```python
from build123d import *

# Parameters (mm, degrees)
SKETCH1_W           = 220
SKETCH1_H           = 30
BOSS_EXTRUDE1_DEPTH = 5
SKETCH2_W           = 30
SKETCH2_H           = 70
BOSS_EXTRUDE2_DEPTH = 5
CUT_EXTRUDE1_DEPTH  = 10
BOSS_EXTRUDE3_DEPTH = 5
BOSS_EXTRUDE4_DEPTH = 30
FILLET1_R           = 5
SKETCH7_R           = 7.5
CUT_EXTRUDE2_DEPTH  = 253
SKETCH8_W           = 15
SKETCH8_H           = 14.618243145
BOSS_EXTRUDE5_DEPTH = 5
FILLET2_R           = 5
CUT_EXTRUDE3_DEPTH  = 5
SKETCH10_W          = 5.944140112
SKETCH10_H          = 11.167837108
SKETCH10_W_2        = 5.92832961
SKETCH10_H_2        = 9.506983552
CUT_EXTRUDE4_DEPTH  = 5
SKETCH11_W          = 5.623434756
SKETCH11_H          = 8.337110403
SKETCH11_W_2        = 5.64698147
SKETCH11_H_2        = 9.10404701
CUT_EXTRUDE5_DEPTH  = 5
FILLET3_R           = 1
CUT_EXTRUDE6_DEPTH  = 5
SKETCH13_W          = 6.176524638
SKETCH13_H          = 11.481735796
SKETCH13_W_2        = 6.413794009
SKETCH13_H_2        = 10.832022022
CUT_EXTRUDE7_DEPTH  = 5


with BuildPart() as part:
    # Sketch1 → Boss-Extrude1 (new body)
    with BuildSketch(Plane(origin=(0, 0, 0), x_dir=(1, 0, 0), z_dir=(0, 1, 0))):
        Rectangle(SKETCH1_W, SKETCH1_H)
    extrude(amount=BOSS_EXTRUDE1_DEPTH)

    # Sketch2 → Boss-Extrude2 (add)
    with BuildSketch(Plane.ZY.offset(110)):
        with Locations((0, -30)):
            Rectangle(SKETCH2_W, SKETCH2_H)
    boss_extrude2 = extrude(amount=BOSS_EXTRUDE2_DEPTH)

    # Mirror1: Boss-Extrude2 across plane
    add(boss_extrude2.mirror(Plane(origin=(0, 0, 0), x_dir=(0, 0, 1), z_dir=(1, 0, 0))))

    # Sketch4 → Cut-Extrude1 (cut)
    with BuildSketch(Plane.ZY.offset(115)):
        with BuildLine():
            Line((-15, -47.167473829), (-15, -65))
            Line((-15, -65), (15, -65))
            Line((15, -65), (15, -47.167473829))
            ThreePointArc((15, -47.167473829), (0, -62.167473829), (-15, -47.167473829))
        make_face()
    cut_extrude1 = extrude(amount=-CUT_EXTRUDE1_DEPTH, mode=Mode.SUBTRACT)

    # Mirror2: Cut-Extrude1 across plane
    add(cut_extrude1.mirror(Plane(origin=(0, 0, 0), x_dir=(0, 0, 1), z_dir=(1, 0, 0))), mode=Mode.SUBTRACT)

    # Sketch5 → Boss-Extrude3 (add)
    with BuildSketch(Plane(origin=(115, 0, 0), x_dir=(0, 0, -1), z_dir=(1, 0, 0))):
        with BuildLine():
            Line((28.523256762, -29.22115135), (15, -31.288780588))
            Line((15, -31.288780588), (-5.201478884, -40.890888071))
            Line((-5.201478884, -40.890888071), (-4.123987776, -59.07486744))
            Line((-4.123987776, -59.07486744), (0, -62.167473829))
            ThreePointArc((0, -62.167473829), (7.341637998, -60.248007132), (12.804338712, -54.98085403))
            Line((12.804338712, -54.98085403), (28.523256762, -29.22115135))
        make_face()
    boss_extrude3 = extrude(amount=-BOSS_EXTRUDE3_DEPTH)

    # Mirror3: Boss-Extrude3 across plane
    add(boss_extrude3.mirror(Plane(origin=(0, 0, 0), x_dir=(0, 0, 1), z_dir=(1, 0, 0))))

    # Sketch6 → Boss-Extrude4 (add, symmetric)
    with BuildSketch(Plane(origin=(0, 0, 0), x_dir=(0, 0, -1), z_dir=(1, 0, 0))):
        Polygon((12.470905957, 5), (35.245651902, 5), (80.752027939, -26.036386601), (77.934766812, -30.167129844), (33.702918166, 0), (12.470905957, 0), align=None)
    extrude(amount=BOSS_EXTRUDE4_DEPTH, both=True)

    # Fillet1
    fillet1_edges = [part.edges().sort_by_distance(p)[0] for p in [
        (-112.5, -31.288780588, -15),
        (0, 5, -35.245651902),
        (-30, 2.5, -15),
        (0, 0, -33.702918166),
        (30, 2.5, -15),
        (-115, 5, 0),
        (115, 5, 0),
        (-110, 0, 0),
        (110, 0, 0),
        (112.5, -31.288780588, -15),
    ]]
    fillet(fillet1_edges, radius=FILLET1_R)

    # Sketch7 → Cut-Extrude2 (cut)
    with BuildSketch(Plane.ZY.offset(115)):
        with Locations((0, -47.167473829)):
            Circle(SKETCH7_R)
    extrude(amount=-CUT_EXTRUDE2_DEPTH, mode=Mode.SUBTRACT)

    # Sketch8 → Boss-Extrude5 (add)
    with BuildSketch(Plane.XY.offset(15)):
        with Locations((-107.5, -39.858352256)):
            Rectangle(SKETCH8_W, SKETCH8_H)
        with Locations((107.5, -39.858352256)):
            Rectangle(SKETCH8_W, SKETCH8_H)
    extrude(amount=BOSS_EXTRUDE5_DEPTH)

    # Fillet2
    fillet2_edges = [part.edges().sort_by_distance(p)[0] for p in [
        (100, -47.167473829, 17.5),
        (100, -32.549230684, 17.5),
        (112.5, -32.549230684, 15),
        (112.5, -47.167473829, 15),
        (-100, -47.167473829, 17.5),
        (-100, -32.549230684, 17.5),
        (-112.5, -47.167473829, 15),
        (-112.5, -32.549230684, 15),
    ]]
    fillet(fillet2_edges, radius=FILLET2_R - 0.0001)  # a hair under: the kernel refuses the full size

    # Sketch9 → Cut-Extrude3 (cut)
    with BuildSketch(Plane(origin=(0, 5, 0), x_dir=(1, 0, 0), z_dir=(0, 1, 0))):
        with BuildLine():
            Line((-77.846940142, 5.680355486), (-57.846940142, 5.680355486))
            Line((-57.846940142, 5.680355486), (57.752992387, 6))
            Line((57.752992387, 6), (77.752992387, 6))
            ThreePointArc((77.752992387, 6), (83.752992387, 0), (77.752992387, -6))
            Line((77.752992387, -6), (57.752992387, -6))
            Line((57.752992387, -6), (-57.846940142, -6.319644514))
            Line((-57.846940142, -6.319644514), (-77.846940142, -6.319644514))
            ThreePointArc((-77.846940142, -6.319644514), (-83.846940142, -0.319644514), (-77.846940142, 5.680355486))
        make_face()
    extrude(amount=-CUT_EXTRUDE3_DEPTH, mode=Mode.SUBTRACT)

    # Sketch10 → Cut-Extrude4 (cut)
    with BuildSketch(Plane(origin=(0, 5, 0), x_dir=(1, 0, 0), z_dir=(0, 1, 0))):
        with Locations((-77.032885662, 7.498184757)):
            Rectangle(SKETCH10_W, SKETCH10_H)
        with Locations((59.124549755, 8.599122626)):
            Rectangle(SKETCH10_W_2, SKETCH10_H_2)
    extrude(amount=-CUT_EXTRUDE4_DEPTH, mode=Mode.SUBTRACT)

    # Sketch11 → Cut-Extrude5 (cut)
    with BuildSketch(Plane(origin=(0, 5, 0), x_dir=(1, 0, 0), z_dir=(0, 1, 0))):
        with Locations((76.926952234, -8.270502887)):
            Rectangle(SKETCH11_W, SKETCH11_H)
        with Locations((-59.100127848, -7.887034583)):
            Rectangle(SKETCH11_W_2, SKETCH11_H_2)
    extrude(amount=-CUT_EXTRUDE5_DEPTH, mode=Mode.SUBTRACT)

    # Fillet3
    fillet3_edges = [part.edges().sort_by_distance(p)[0] for p in [
        (-80.004955718, 2.5, -5.278834634),
        (62.08871456, 2.5, -6),
        (56.16038495, 2.5, -5.995596293),
        (-74.060815606, 2.5, -5.680355486),
        (-61.923618583, 2.5, 6.319644514),
        (-56.276637113, 2.5, 6.31530248),
        (74.115234856, 2.5, 6),
        (79.738669612, 2.5, 5.661897735),
    ]]
    fillet(fillet3_edges, radius=FILLET3_R)

    # Sketch12 → Cut-Extrude6 (cut)
    with BuildSketch(Plane(origin=(0, 19.819293064, -13.51721001), x_dir=(1, 0, 0), z_dir=(0, 0.8261486486486485, -0.563452225424669))):
        with BuildLine():
            Line((13.839167564, 62.402963996), (-12.615635754, 62.402963996))
            ThreePointArc((-12.615635754, 62.402963996), (-18.615635754, 68.402963996), (-12.615635754, 74.402963996))
            Line((-12.615635754, 74.402963996), (13.839167564, 74.402963996))
            ThreePointArc((13.839167564, 74.402963996), (19.839167564, 68.402963996), (13.839167564, 62.402963996))
        make_face()
    extrude(amount=-CUT_EXTRUDE6_DEPTH, mode=Mode.SUBTRACT)

    # Sketch13 → Cut-Extrude7 (cut)
    with BuildSketch(Plane(origin=(0, 19.819293064, -13.51721001), x_dir=(1, 0, 0), z_dir=(0, 0.8261486486486485, -0.563452225424669))):
        with Locations((8.803081479, 59.323306986)):
            Rectangle(SKETCH13_W, SKETCH13_H)
        with Locations((-8.792921623, 58.998450099)):
            Rectangle(SKETCH13_W_2, SKETCH13_H_2)
    extrude(amount=-CUT_EXTRUDE7_DEPTH, mode=Mode.SUBTRACT)


solid = part.part
```
Can you work these out from the model? Positions are in its coordinate system, mm. A direction names the side the tool comes from. Coordinates: 2 decimals unless noted, no trailing zeros. Loops run counter-clockwise (first coordinate to the right, second up) from the corner with the lowest first, then second, coordinate; pieces in that order, holes last. Notation, with made-up numbers: (-20, 66.5) - (25, 66.5) arc R13 cw to (25, 88.5) - close; hole circle Ø11 at (-36, 40). An arc over 180 degrees is marked (long way). Use a Markdown table: item, result.
Item 1: For faces 1 (the face through (8.8, -12.4, -56.4)), 2 (the face through (79.739, 3, 9)), 3 (the face through (-1, 0, -9)), 4 (the face through (112.46, -29.22, -16.7)), 5 (the face through (100, -40, 17)), which set-ups out of +Z, -Z, +X, -X, +Y, -Y let a thin tool reach every point of the face, with its end or its side?
Numbers:
| item | result |
|---|---|
| face 1 | -Z, -Y |
| face 2 | +Y, -Y |
| face 3 | +Z, -Y |
| face 4 | +X, -X, +Y |
| face 5 | +Z, -Z, +Y, -Y |
Item 2: We'd pull the mould along X, two halves only. Please class faces 6 (the face through (-113, 4, 0)), 7 (the face through (-61.924, 3, 10)), 8 (the face through (30, -10, -51)): released by +X, released by -X, zero draft, split by the parting line, or undercut.
Numbers:
| item | result |
|---|---|
| face 6 | released by -X |
| face 7 | undercut |
| face 8 | released by +X |
Item 3: Will these pins go through, and if not, where does the flat tip stop? pin 1 (1 mm diameter, centred on x = -12, y = -13, fed in from -Z); pin 2 (4 mm diameter, centred on y = 1.5, z = 9, fed in from -X); pin 3 (1.5 mm diameter, centred on y = 3, z = -8.5, fed in from -X); pin 4 (5.5 mm diameter, centred on x = 111, z = 16.5, fed in from -Y).
Numbers:
| item | result |
|---|---|
| pin 1 | stops at z = -62.37 |
| pin 2 | stops at x = -115 |
| pin 3 | stops at x = -114.47 |
| pin 4 | stops at y = -53.16 |
Item 4: I want a section at A-A on x = -44.5. Please give me the cut outline in (y, z).
Numbers:
| item | result |
|---|---|
| outline | (0, -15) - (5, -15) - (5, -5.72) - (0, -5.72) - close; (0, 6.28) - (5, 6.28) - (5, 15) - (0, 15) - close |
Item 5: If I drill on probe 1 along X at (y, z) = (-49, 13.5); probe 2 along Y at (x, z) = (112.7, 0); probe 3 along X at (y, z) = (-7.5, -53.5), over which ranges is the centre line in solid material (lowest first)? Write a range as from..to.
Numbers:
| item | result |
|---|---|
| probe 1 | x = -115..-110, 110..115 |
| probe 2 | y = -62.17..-54.67, -39.67..4.21 |
| probe 3 | x = -30..30 |
